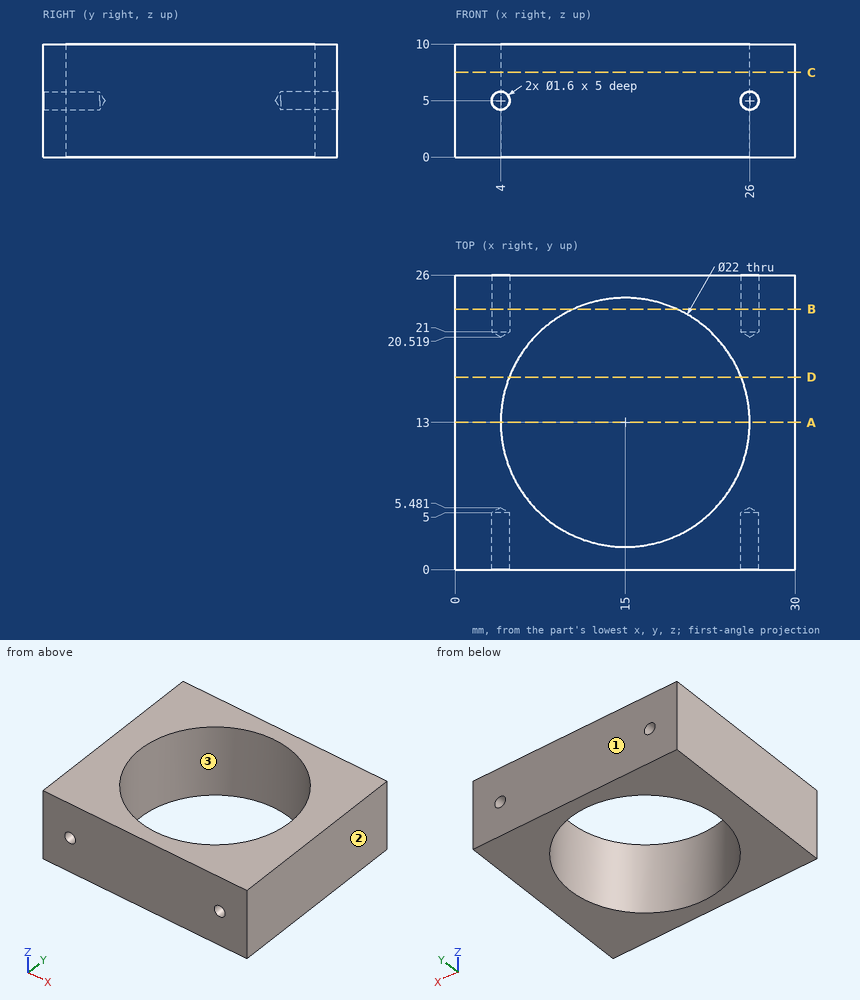
Print and shaded views of the part. All mm, measured from the part's lowest x, y and z. Coordinates: 2 decimals unless noted, no trailing zeros. Write each loop counter-clockwise with the first axis right and the second up, starting at its lowest first coordinate (ties: lowest second). Pieces come first, ordered by that corner, then holes. Notation, with made-up numbers: (69.5, 45) - (107.5, 45) arc R14 ccw to (107.5, 69) - close; hole circle Ø10 at (20.25, -28). An arc over 180 degrees is marked (long way). One line per question, with ' | ' between items. Start each with the question number.
Q1. Drill centre lines: line 1 (Y direction, x = 15.25, z = 6); line 2 (X direction, y = 1.6, z = 5); line 3 (Z direction, x = 26, y = 23.65). Where is each one in solid material? Low to high. Write a range as [from, to].
Q2. Cut at D-D, the plane y = 17. List the corners of the cut face in (x, z).
Q3. Pin check, flat tips, straight feed: pin 1 (4 mm diameter, centred on x = 8, y = 10, fed in from +Z); pin 2 (1 mm diameter, centred on x = 4, z = 5, fed in from -Y). Stop position of each tip, or through.
Q4. Pull direction Y, two halves, no side cores. Call the marked faces 1, 2 and 3: pulls with the +Y half, pulls with the -Y half, needs draft (parallel to the pull), parting line crosses it, or undercut.
Q5. Cut at A-A, the plane y = 13. List the corners of the cut face in (x, z).
Q6. Cut at C-C, the plane z = 7.5. List the corners of the cut face in (x, y), then the cut area to 3 significant figures.
Q7. Cut at B-B, the plane y = 23. List the corners of the cut face in (x, z).
Answer below:
1) line 1: [0, 2], [24, 26] | line 2: [0, 3.2], [4.8, 25.2], [26.8, 30] | line 3: [0, 4.2], [5.8, 10]
2) outline: (0, 0) - (4.75, 0) - (4.75, 10) - (0, 10) - close; (25.25, 0) - (30, 0) - (30, 10) - (25.25, 10) - close
3) pin 1: through | pin 2: y = 5.18
4) face 1: pulls with the +Y half | face 2: needs draft | face 3: undercut
5) outline: (0, 0) - (4, 0) - (4, 10) - (0, 10) - close; (26, 0) - (30, 0) - (30, 10) - (26, 10) - close
6) outline: (0, 0) - (30, 0) - (30, 26) - (0, 26) - close; hole circle Ø22 at (15, 13) | area: 400 mm^2
7) outline: (0, 0) - (10.42, 0) - (10.42, 10) - (0, 10) - close; (19.58, 0) - (30, 0) - (30, 10) - (19.58, 10) - close; hole circle Ø1.6 at (4, 5); hole circle Ø1.6 at (26, 5)
